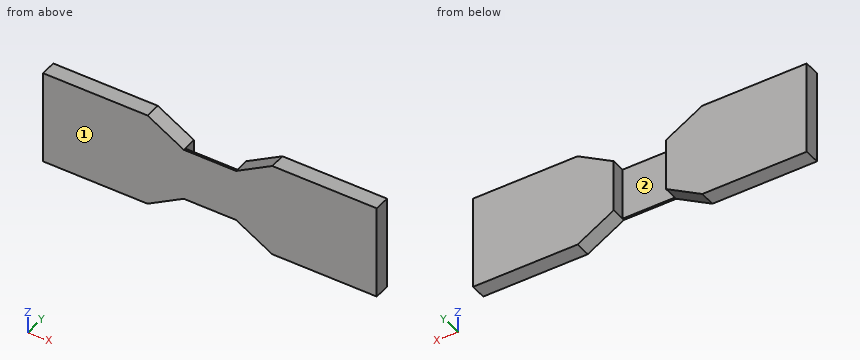
from build123d import *

# Parameters (mm, degrees)
BOSS_EXTRUDE1_DEPTH   = 3
BOSS_EXTRUDE1_2_DEPTH = 3
SKETCH1_3_W           = 10
SKETCH1_3_H           = 10
BOSS_EXTRUDE2_DEPTH   = 0.4


with BuildPart() as part:
    # Sketch1 → Boss-Extrude1 (new body)
    with BuildSketch(Plane(origin=(0, 0, 0), x_dir=(1, 0, 0), z_dir=(0, 1, 0))):
        Polygon((-10, 5.029673591), (-10, -4.970326409), (-16.92820323, -8.970326409), (-36.92820323, -8.970326409), (-36.92820323, 9.029673591), (-16.92820323, 9.029673591), align=None)
    extrude(amount=BOSS_EXTRUDE1_DEPTH)



with BuildPart() as body_2:
    # Sketch1 → Boss-Extrude1 2 (new body)
    with BuildSketch(Plane(origin=(0, 0, 0), x_dir=(1, 0, 0), z_dir=(0, 1, 0))):
        Polygon((0, 5.029673591), (6.92820323, 9.029673591), (26.92820323, 9.029673591), (26.92820323, -8.970326409), (6.92820323, -8.970326409), (0, -4.970326409), align=None)
    extrude(amount=BOSS_EXTRUDE1_2_DEPTH)


with BuildPart() as part_1:
    add(part.part)

    add(body_2.part)  # Boss-Extrude2 merges body 2
    # Sketch1_3 → Boss-Extrude2 (add)
    with BuildSketch(Plane(origin=(0, 0, 0), x_dir=(1, 0, 0), z_dir=(0, 1, 0))):
        with Locations((-5, 0.029673591)):
            Rectangle(SKETCH1_3_W, SKETCH1_3_H)
    extrude(amount=BOSS_EXTRUDE2_DEPTH)


solid = part_1.part
CAD build for the part. Positions are in the model's coordinates, mm. Face numbers are marked on the shaded views. Round coordinates to 2 decimals unless told otherwise and drop trailing zeros. Write each loop counter-clockwise with the first axis right and the second up, starting at its lowest first coordinate (ties: lowest second). Pieces come first, ordered by that corner, then holes. Notation, with made-up numbers: M -4,40.25 L 0,40.25 A21 ccw 0,44.25 Z; hole C -38,-16.75 d6. An arc over 180 degrees is marked long. Put each result on its own line as item: value. Start each with the question number.
1) Pull direction X, two halves, no side cores. Call the marked faces 1 and 2: pulls with the +X half, pulls with the -X half, needs draft (parallel to the pull), parting line crosses it, or undercut.
2) Saw through at A-A, the plane y = 1.4. Write the cut outline in (x, z), and give its area (3 significant figures).
3) Saw through at C-C, the plane z = 0.25. Write the cut outline in (x, y).
4) Saw through at B-B, the plane z = 5.75. Write the cut outline in (x, y), and give its area (3 significant figures).
5) Saw through at D-D, the plane x = 3. Write the cut outline in (y, z).
6) Drill centre lines: probe 1 along X at (y, z) = (1.8, -4); probe 2 along Z at (x, y) = (-1, 0.25); probe 3 along Y at (x, z) = (-2, 0). Where is each one in solid material? Low to high. Write a range as [from, to].
Resolved:
1. face 1: needs draft
1. face 2: undercut
2. outline: M -36.93,-9.03 L -16.93,-9.03 L -10,-5.03 L -10,4.97 L -16.93,8.97 L -36.93,8.97 Z; M 0,-5.03 L 6.93,-9.03 L 26.93,-9.03 L 26.93,8.97 L 6.93,8.97 L 0,4.97 Z
2. area: 914 mm²
3. outline: M -36.93,0 L 26.93,0 L 26.93,3 L 0,3 L 0,0.4 L -10,0.4 L -10,3 L -36.93,3 Z
4. outline: M -36.93,0 L -11.35,0 L -11.35,3 L -36.93,3 Z; M 1.35,0 L 26.93,0 L 26.93,3 L 1.35,3 Z
4. area: 153 mm²
5. outline: M 0,-6.76 L 3,-6.76 L 3,6.7 L 0,6.7 Z
6. probe 1: [-36.93, -10], [0, 26.93]
6. probe 2: [-5.03, 4.97]
6. probe 3: [0, 0.4]
